from build123d import *

# Parameters (mm, degrees)
BOSS_EXTRUDE1_DEPTH = 5
CUT_EXTRUDE1_DEPTH  = 2
SKETCH3_R           = 10
CUT_EXTRUDE2_DEPTH  = 9
SKETCH4_R           = 15
SKETCH4_R_2         = 10
BOSS_EXTRUDE2_DEPTH = 2


with BuildPart() as part:
    # Sketch1 → Boss-Extrude1 (new body, symmetric)
    with BuildSketch(Plane(origin=(0, 0, 0), x_dir=(1, 0, 0), z_dir=(0, 1, 0))):
        with BuildLine():
            ThreePointArc((14.41480993, 54.148885958), (-2.094976259, 64.852982006), (-15, 50))
            Line((-15, 50), (-30, 0))
            ThreePointArc((-30, 0), (0, -30), (30, 0))
            Line((30, 0), (14.41480993, 54.148885958))
        make_face()
    extrude(amount=BOSS_EXTRUDE1_DEPTH, both=True)

    # Sketch2 → Cut-Extrude1 (cut)
    with BuildSketch(Plane(origin=(0, 5, 0), x_dir=(1, 0, 0), z_dir=(0, 1, 0))):
        with BuildLine():
            Line((24.99092108, -0.673693969), (9.609873286, 52.765923972))
            ThreePointArc((9.609873286, 52.765923972), (-1.723304272, 59.850391992), (-9.978133058, 49.339045626))
            Line((-9.978133058, 49.339045626), (-24.990168055, -0.701071031))
            ThreePointArc((-24.990168055, -0.701071031), (0.013693708, -24.99999625), (24.99092108, -0.673693969))
        make_face()
    cut_extrude1 = extrude(amount=-CUT_EXTRUDE1_DEPTH, mode=Mode.SUBTRACT)

    # Mirror1: Cut-Extrude1 across plane
    add(cut_extrude1.mirror(Plane.ZX), mode=Mode.SUBTRACT)

    # Sketch3 → Cut-Extrude2 (cut, through all)
    with BuildSketch(Plane(origin=(0, 3, 0), x_dir=(1, 0, 0), z_dir=(0, 1, 0))):
        Circle(SKETCH3_R)
    extrude(amount=-CUT_EXTRUDE2_DEPTH, mode=Mode.SUBTRACT)

    # Sketch4 → Boss-Extrude2 (add)
    with BuildSketch(Plane(origin=(0, 3, 0), x_dir=(1, 0, 0), z_dir=(0, 1, 0))):
        Circle(SKETCH4_R)
        Circle(SKETCH4_R_2, mode=Mode.SUBTRACT)
    boss_extrude2 = extrude(amount=BOSS_EXTRUDE2_DEPTH)

    # Mirror2: Boss-Extrude2 across plane
    add(boss_extrude2.mirror(Plane.ZX))


solid = part.part
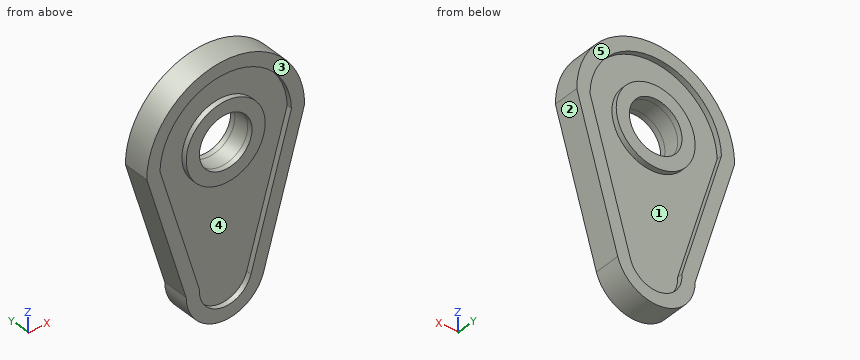
Design review of the part built by this model. Coordinates are the model's own, in mm. Face numbers are marked on the shaded views. A direction names the side the tool comes from. Give positions to 0.01 mm unless a question says otherwise; leave off trailing zeros. Loops run counter-clockwise (first coordinate to the right, second up) from the corner with the lowest first, then second, coordinate; pieces in that order, holes last. Notation, with made-up numbers: (-13.75, 8.5) - (-4.75, 8.5) arc R21 cw to (-4.75, 13.5) - close; hole circle Ø5 at (-13, -24). An arc over 180 degrees is marked (long way). Use CSV: the item, a comma, the result in double quotes. Start each with the question number.
1. Add section D-D (z = -45). State the section outline as (x, y) points.
2. Add section A-A (x = -4.5). State the section outline as (y, z) points, plus the area to 3 significant figures.
3. Draft analysis for pull direction X (two halves, no side actions). For the marked faces 1, 2 and 3, state which applies: released by +X, released by -X, zero draft, split by the parting line, or undercut.
4. Add section B-B (z = 3). State the section outline as (x, y) points.
5. Insertion check: P1, Ø2, axis at x = -6, z = -15, coming from the +Y side; P2, Ø1.5, axis at y = -2.5, z = -3.5, coming from the +X side; P3, Ø3, axis at x = 8.5, y = -2, coming from the -Z side; P4, Ø12, axis at x = 0, z = 0, coming from the +Y side. Each pin has a flat end and moves straight along its axis. Give the tip position at first contact, or say it passes through.
6. Add section C-C (y = 0.5). State the section outline as (x, z) points.
7. Wall thickness on L1, parallel to Z at x = 0, y = 4.5; L2, parallel to Z at x = 0, y = 1.65; L3, parallel to X at y = 3.25, z = -9: over which ranges is each line inside the solid? List them lowest first.
8. Machinability: for the marked faces 4 and 5, which of the approach directions +Z, -Z, +X, -X, +Y, -Y give a long, thin tool a straight path to every point of the face, cutting with its end or side? Answer none if there is none.
Results found:
1,outline,"(-16.5, -5) - (-11.28, -5) - (-11.28, -3) - (11.85, -3) - (11.85, -5) - (17.05, -5) - (17.05, 5) - (11.85, 5) - (11.85, 3) - (-11.28, 3) - (-11.28, 5) - (-16.5, 5) - close"
2,outline,"(-5, -64.31) - (5, -64.31) - (5, -58.93) - (3, -58.93) - (3, -14.31) - (5, -14.31) - (5, -8.93) - (-5, -8.93) - (-5, -14.31) - (-3, -14.31) - (-3, -58.93) - (-5, -58.93) - close; (-5, 8.93) - (5, 8.93) - (5, 14.31) - (3, 14.31) - (3, 24.59) - (5, 24.59) - (5, 29.66) - (-5, 29.66) - (-5, 24.59) - (-3, 24.59) - (-3, 14.31) - (-5, 14.31) - close"
2,area,"541 mm²"
3,face 1,"undercut"
3,face 2,"released by +X"
3,face 3,"zero draft"
4,outline,"(-29.85, -5) - (-24.82, -5) - (-24.82, -3) - (-14.7, -3) - (-14.7, -5) - (-9.54, -5) - (-9.54, 5) - (-14.7, 5) - (-14.7, 3) - (-24.82, 3) - (-24.82, 5) - (-29.85, 5) - close; (9.54, -5) - (14.7, -5) - (14.7, -3) - (24.82, -3) - (24.82, -5) - (29.85, -5) - (29.85, 5) - (24.82, 5) - (24.82, 3) - (14.7, 3) - (14.7, 5) - (9.54, 5) - close"
5,P1,"stops at y = 3"
5,P2,"stops at x = 29.21"
5,P3,"stops at z = -63.27"
5,P4,"passes through"
6,outline,"(-30, 0) - (-15, -50) arc R15 ccw to (14.41, -54.15) - (30, 0) arc R30 ccw to start; hole circle Ø20 at (0, 0)"
7,L1,"z = -65 to -60, -15 to -10, 10 to 15, 25 to 30"
7,L2,"z = -65 to -10, 10 to 30"
7,L3,"x = -27.3 to -22.08, -12 to -4.36, 4.36 to 12, 22.21 to 27.41"
8,face 4,"-Y"
8,face 5,"+Z, -Z, +X, -X, +Y"
